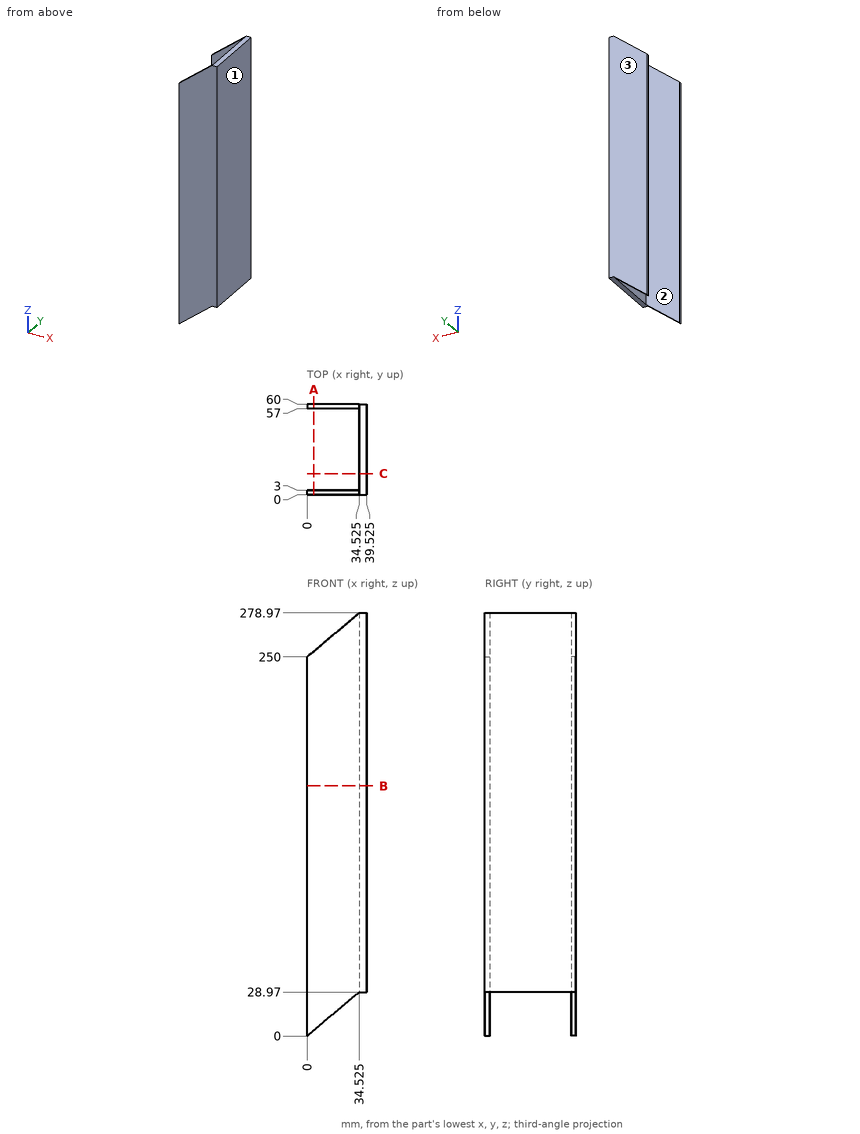
Geometry check sheet. Reference: drawing and pictorial views, mm from the part's lowest x, y, z. Round coordinates to 2 decimals unless told otherwise and drop trailing zeros. Loops run counter-clockwise (first coordinate to the right, second up) from the corner with the lowest first, then second, coordinate; pieces in that order, holes last.
1. Gauge pin test, flat ends, axial feed: pin 1 Ø12 at (x, y) = (4, 47) entering from -Z; pin 2 Ø1.5 at (x, y) = (37.5, 40) entering from -Z; pin 3 Ø12 at (y, z) = (23.5, 250) entering from -X (3 decimals). Record the tip position at first contact, or that the pin passes through.
2. Sectioned sample at B-B on z = 165. Record the boundary of the cut face in (x, y) (1 decimal).
3. Mould release check, pull along Y, two halves, no side actions. Record for the marked faces 1, 2 and 3: released by +Y, released by -Y, zero draft, split by the parting line, or undercut.
4. Scan lines: probe 1 along Y at (x, z) = (31, 213); probe 2 along X at (y, z) = (51, 261.5) (1 decimal); probe 3 along Z at (x, y) = (36, 33). Record each from-to range of solid material in increasing order.
5. Sectioned sample at A-A on x = 4.5. Record the boundary of the cut face in (y, z), and give its area (3 significant figures).
6. Sectioned sample at C-C on y = 14. Record the boundary of the cut face in (x, z) (1 decimal), and give its area (3 significant figures).
Recorded:
1. pin 1: passes through
1. pin 2: stops at z = 28.97
1. pin 3: stops at x = 34.525
2. outline: (0, 0) - (39.5, 0) - (39.5, 60) - (0, 60) - (0, 57) - (34.5, 57) - (34.5, 3) - (0, 3) - close
3. face 1: zero draft
3. face 2: undercut
3. face 3: released by +Y
4. probe 1: y = 0 to 3, 57 to 60
4. probe 2: x = 34.5 to 39.5
4. probe 3: z = 28.97 to 278.97
5. outline: (0, 3.78) - (3, 3.78) - (3, 253.78) - (0, 253.78) - close; (57, 3.78) - (60, 3.78) - (60, 253.78) - (57, 253.78) - close
5. area: 1,500 mm2
6. outline: (34.5, 29) - (39.5, 29) - (39.5, 279) - (34.5, 279) - close
6. area: 1,250 mm2
